Source: CAD feature listing. Evaluate the final solid. Frame: model axes, mm. Face numbers are marked on the shaded views. A direction names the side the tool comes from. Round coordinates to 2 decimals unless told otherwise and drop trailing zeros. Order: outer loops, then holes, each group sorted by start corner. A loop starts at its lowest first (then second) coordinate and runs counter-clockwise, first axis right, second up. Notation, with made-up numbers: (67, 83) -> (88, 83) arc R16 cw to (88, 105) -> close; hole circle Ø5 at (72, -1.75). An arc over 180 degrees is marked (long way). Write item = value, one per line. Start each with the question number.
(1) Cut plane A-A on x = 38.1. Return the cut outline in (y, z), then the cut area to 4 significant figures.
(2) Reachability of the marked faces 4 and 5 from +Z, -Z, +X, -X, +Y, -Y: full face, straight path, thin tool, end or side. Return the list, or none.
(3) Cut plane B-B on y = 12.7. Return the cut outline in (x, z).
(4) Contact query for flat-ended pins moving along their axis: pin 1 Ø9.5 at (x, y) = (63.5, 12.7) entering from -Z; pin 2 Ø13 at (x, y) = (11, 13) entering from +Z; pin 3 Ø9.5 at (x, y) = (40.5, 13) entering from +Z; pin 4 Ø8 at (x, y) = (63.5, 12.7) entering from +Z. Output: stop coordinate, or through.
(5) Draft query along Z for the marked faces 1, 2 and 3. Return one class per face: released by +Z, released by -Z, zero draft, split by the parting line, or undercut.
(6) Cut plane D-D on y = 19.5. Return the cut outline in (x, z).
(7) Cut plane C-C on z = 27. Return the cut outline in (x, y), then the cut area to 3 significant figures.
(8) Ray query, line 1 (X direction, y = 6.5, z = 21); line 2 (X direction, y = 8.75, z = 21); line 3 (Y direction, x = 12.7, z = 19.25). Return the intervals inside material, ascending.
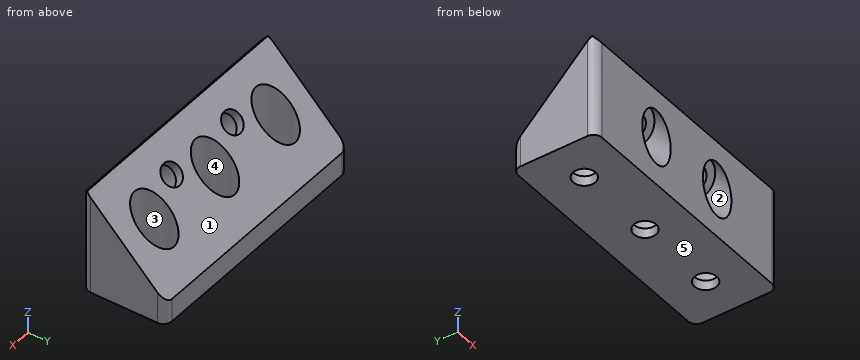
from build123d import *

# Parameters (mm, degrees)
SKETCH3_W                                        = 76.2
SKETCH3_H                                        = 25.4
BOSS_EXTRUDE1_DEPTH                              = 31.75
CBORE_FOR_1_4_BUTTON_HEAD_CAP_SCREW1_D           = 6.7564
CBORE_FOR_1_4_BUTTON_HEAD_CAP_SCREW1_CBORE_D     = 11.90752
CBORE_FOR_1_4_BUTTON_HEAD_CAP_SCREW1_CBORE_DEPTH = 28.7528
CUT_EXTRUDE1_START                               = -76.2
CUT_EXTRUDE1_DEPTH                               = 76.2
CBORE_FOR_1_4_BUTTON_HEAD_CAP_SCREW2_D           = 6.7564
CBORE_FOR_1_4_BUTTON_HEAD_CAP_SCREW2_CBORE_D     = 11.90752
CBORE_FOR_1_4_BUTTON_HEAD_CAP_SCREW2_CBORE_DEPTH = 22.4028
FILLET1_R                                        = 2.54


# Read off the part's stored shape, not the designer's step: Cut-Extrude1
with BuildPart() as part:
    # Sketch3 → Boss-Extrude1 (new body)
    with BuildSketch(Plane.XY):
        with Locations((38.1, 12.7)):
            Rectangle(SKETCH3_W, SKETCH3_H)
    extrude(amount=BOSS_EXTRUDE1_DEPTH)

    # CBORE for 1/4 Button Head Cap Screw1 (through all)
    with Locations(Plane.XY.offset(31.75)):
        with Locations((12.7, 12.7), (38.1, 12.7), (63.5, 12.7)):
            CounterBoreHole(CBORE_FOR_1_4_BUTTON_HEAD_CAP_SCREW1_D / 2, CBORE_FOR_1_4_BUTTON_HEAD_CAP_SCREW1_CBORE_D / 2, CBORE_FOR_1_4_BUTTON_HEAD_CAP_SCREW1_CBORE_DEPTH)

    # Cut-Extrude1 outline → Cut-Extrude1 (cut)
    with BuildSketch(Plane(origin=(76.2, 0, 0), x_dir=(0, 0, -1), z_dir=(1, 0, 0)).offset(CUT_EXTRUDE1_START)):
        Polygon((-31.75, 0), (-29.761484683, 0), (-31.080742341, 1.319257659), (-7, 25.4), (-31.75, 25.4), align=None)
    extrude(amount=CUT_EXTRUDE1_DEPTH, mode=Mode.SUBTRACT)

    # CBORE for 1/4 Button Head Cap Screw2 (through all)
    with Locations(Plane(origin=(0, -1.760512242, -1.760512242), x_dir=(1, 0, 0), z_dir=(0, -0.7071067811865437, -0.7071067811865513))):
        with Locations((25.4, 10.522273819), (50.8, 10.522273819)):
            CounterBoreHole(CBORE_FOR_1_4_BUTTON_HEAD_CAP_SCREW2_D / 2, CBORE_FOR_1_4_BUTTON_HEAD_CAP_SCREW2_CBORE_D / 2, CBORE_FOR_1_4_BUTTON_HEAD_CAP_SCREW2_CBORE_DEPTH)

    # Fillet1
    fillet1_edges = [part.edges().sort_by_distance(p)[0] for p in [
        (0, 0, 14.880742341),
        (0, 25.4, 3.5),
        (76.2, 25.4, 3.5),
        (76.2, 0, 14.880742341),
    ]]
    fillet(fillet1_edges, radius=FILLET1_R)


solid = part.part
Evaluation:
q1.outline = (0, 0) -> (9.32, 0) -> (9.32, 3) -> (6.75, 3) -> (6.75, 25.65) -> (1.32, 31.08) -> (0, 29.76) -> close; (16.08, 0) -> (25.4, 0) -> (25.4, 7) -> (18.65, 13.75) -> (18.65, 3) -> (16.08, 3) -> close
q1.area = 279.5 mm^2
q2.face_4 = +Z
q2.face_5 = -Z, +X, -X, +Y, -Y
q3.outline = (0, 0) -> (9.32, 0) -> (9.32, 3) -> (6.75, 3) -> (6.75, 19.7) -> (0, 19.7) -> close; (16.08, 0) -> (34.72, 0) -> (34.72, 3) -> (32.15, 3) -> (32.15, 19.7) -> (18.65, 19.7) -> (18.65, 3) -> (16.08, 3) -> close; (41.48, 0) -> (60.12, 0) -> (60.12, 3) -> (57.55, 3) -> (57.55, 19.7) -> (44.05, 19.7) -> (44.05, 3) -> (41.48, 3) -> close; (66.88, 0) -> (76.2, 0) -> (76.2, 19.7) -> (69.45, 19.7) -> (69.45, 3) -> (66.88, 3) -> close
q4.pin_1 = 0
q4.pin_2 = 25.9
q4.pin_3 = 23.71
q4.pin_4 = 3
q5.face_1 = released by +Z
q5.face_2 = undercut
q5.face_3 = zero draft
q6.outline = (0, 0) -> (76.2, 0) -> (76.2, 12.9) -> (0, 12.9) -> close
q7.outline = (0, 2.54) arc R2.54 ccw to (2.54, 0) -> (73.66, 0) arc R2.54 ccw to (76.2, 2.54) -> (76.2, 5.4) -> (0, 5.4) -> close
q7.area = 409 mm^2
q8.line_1 = 0 to 19.45, 31.35 to 44.85, 56.75 to 76.2
q8.line_2 = 0 to 8.25, 17.15 to 22.58, 28.22 to 33.65, 42.55 to 47.98, 53.62 to 59.05, 67.95 to 76.2
q8.line_3 = 0 to 6.75
